```python
from build123d import *

# Parameters (mm, degrees)
BOSS_EXTRUDE1_DEPTH = 3
SKETCH2_R           = 2.5
BOSS_EXTRUDE2_DEPTH = 20
SKETCH3_R           = 5
BOSS_EXTRUDE3_DEPTH = 2
SKETCH4_R           = 2.5
BOSS_EXTRUDE4_DEPTH = 18


with BuildPart() as part:
    # Sketch1 → Boss-Extrude1 (new body)
    with BuildSketch(Plane(origin=(0, 0, 0), x_dir=(1, 0, 0), z_dir=(0, 1, 0))):
        with BuildLine():
            Line((-25.769230769, 365.615384615), (-25.769230769, -80.384615385))
            ThreePointArc((-25.769230769, -80.384615385), (-15.769230769, -90.384615385), (-5.769230769, -80.384615385))
            Line((-5.769230769, -80.384615385), (-5.769230769, 365.615384615))
            ThreePointArc((-5.769230769, 365.615384615), (-15.769230769, 375.615384615), (-25.769230769, 365.615384615))
        make_face()
    extrude(amount=BOSS_EXTRUDE1_DEPTH)

    # Sketch2 → Boss-Extrude2 (add)
    with BuildSketch(Plane(origin=(0, 3, 0), x_dir=(1, 0, 0), z_dir=(0, 1, 0))):
        with Locations(Location((-15.769230769, -80.384615385, 0), (0, 0, 90))):
            Circle(SKETCH2_R)
        with Locations(Location((-15.769230769, 365.615384615, 0), (0, 0, 90))):
            Circle(SKETCH2_R)
    extrude(amount=BOSS_EXTRUDE2_DEPTH)

    # Sketch3 → Boss-Extrude3 (add)
    with BuildSketch(Plane.XZ):
        with Locations(Location((-15.769230769, -142.615384615, 0), (0, 0, 270))):
            Circle(SKETCH3_R)
    extrude(amount=BOSS_EXTRUDE3_DEPTH)

    # Sketch4 → Boss-Extrude4 (add)
    with BuildSketch(Plane.XZ.offset(2)):
        with Locations(Location((-15.769230769, -142.615384615, 0), (0, 0, 270))):
            Circle(SKETCH4_R)
    extrude(amount=BOSS_EXTRUDE4_DEPTH)


solid = part.part
```
For this review, take the finished solid that the model builds, in its own axes (mm). A direction names the side the tool comes from. Round coordinates to 2 decimals unless told otherwise and drop trailing zeros. Loops run counter-clockwise (first coordinate to the right, second up) from the corner with the lowest first, then second, coordinate; pieces in that order, holes last.
Q1. Machinability: for faces 1 (the face through (-15.989, 1.479, 90.382)), 2 (the face through (-14.267, -0.986, -147.384)), which of the approach directions +Z, -Z, +X, -X, +Y, -Y give a long, thin tool a straight path to every point of the face, cutting with its end or side? Answer none if there is none.
Result sheet:
face 1: +Z, +Y, -Y
face 2: -Y
Q2. Add section B-B on y = 9. Write out the cut boundary in (x, z).
Result sheet:
outline: circle Ø5 at (-15.77, -365.62); circle Ø5 at (-15.77, 80.38)
Q3. To check wall thickness, follow line 1 along Y through (x, z) = (-20.75, -160.5); line 2 along Z through (x, y) = (-15.25, -11.5); line 3 along Z through (x, y) = (-17.25, 15.5). State the ranges of each line that lie inside material, in increasing order.
Result sheet:
line 1: y = 0 to 3
line 2: z = -145.06 to -140.17
line 3: z = -367.63 to -363.6, 78.37 to 82.4
Q4. Add section A-A on z = -183.5. Write out the cut boundary in (x, y), plus the area to 3 significant figures.
Result sheet:
outline: (-25.77, 0) - (-5.77, 0) - (-5.77, 3) - (-25.77, 3) - close
area: 60.0 mm2
Q5. Insertion check: pin 1 Ø5 at (x, y) = (-18, -13) entering from -Z; pin 2 Ø6 at (x, z) = (-20.5, -180) entering from +Y; pin 3 Ø10 at (x, z) = (-19, -108.5) entering from -Y. Each pin has a flat end and moves straight along its axis. Give the tip position at first contact, or say it passes through.
Result sheet:
pin 1: stops at z = -145.12
pin 2: stops at y = 3
pin 3: stops at y = 0
